Here's how the part is built. I have some questions about the finished solid (model axes, mm). Face numbers are marked on the shaded views. A direction names the side the tool comes from. Round coordinates to 2 decimals unless told otherwise and drop trailing zeros. Write each loop counter-clockwise with the first axis right and the second up, starting at its lowest first coordinate (ties: lowest second). Pieces come first, ordered by that corner, then holes. Notation, with made-up numbers: (69.25, 51) - (78.25, 51) arc R17 ccw to (78.25, 76) - close; hole circle Ø4 at (-39, 19.5). An arc over 180 degrees is marked (long way). Return JSON: item names as keys, results as strings. Group by question number.
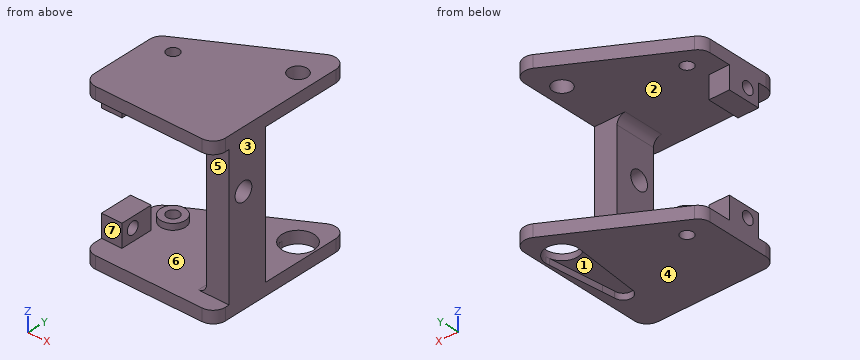
```python
from build123d import *

# Parameters (mm, degrees)
SKETCH1_R           = 1.5
BOSS_EXTRUDE1_DEPTH = 3
SKETCH2_W           = 5
SKETCH2_H           = 8
BOSS_EXTRUDE2_DEPTH = 34
LPATTERN1_COUNT     = 2
LPATTERN1_PITCH     = 37
SKETCH3_W           = 5.5
SKETCH3_H           = 10
BOSS_EXTRUDE4_DEPTH = 34
SKETCH5_W           = 23
SKETCH5_H           = 8
CUT_EXTRUDE1_DEPTH  = 10
CUT_EXTRUDE11_START = -3.7
SKETCH9_R           = 1.5
CUT_EXTRUDE11_DEPTH = 2.2
SKETCH11_R          = 3
SKETCH11_R_2        = 1.5
BOSS_EXTRUDE5_DEPTH = 1.5
SKETCH12_R          = 1.5
CUT_EXTRUDE13_DEPTH = 62.719864532
SKETCH14_R          = 3.9
CUT_EXTRUDE15_DEPTH = 10
SKETCH15_R          = 2.3
CUT_EXTRUDE16_DEPTH = 65.065136212
SKETCH16_R          = 2.25
CUT_EXTRUDE17_DEPTH = 65.065136212
FILLET1_R           = 2


with BuildPart() as part:
    # Sketch1 → Boss-Extrude1 (new body)
    with BuildSketch(Plane.XY):
        with BuildLine():
            Line((-4.5, -2.598076211), (-30.5, -17.60918321))
            ThreePointArc((-30.5, -17.60918321), (-31.598076211, -18.707259422), (-32, -20.207259422))
            Line((-32, -20.207259422), (-32, -35.475208614))
            ThreePointArc((-32, -35.475208614), (-31.121320344, -37.596528958), (-29, -38.475208614))
            Line((-29, -38.475208614), (-3, -38.475208614))
            ThreePointArc((-3, -38.475208614), (-0.878679656, -37.596528958), (0, -35.475208614))
            Line((0, -35.475208614), (0, -5.196152423))
            ThreePointArc((0, -5.196152423), (-1.5, -2.598076211), (-4.5, -2.598076211))
        make_face()
        with Locations((-26, -20.60918321)):
            Circle(SKETCH1_R, mode=Mode.SUBTRACT)
        with Locations((-4.41, -10.598076211)):
            Circle(SKETCH1_R, mode=Mode.SUBTRACT)
    boss_extrude1 = extrude(amount=BOSS_EXTRUDE1_DEPTH)

    # Sketch2 → Boss-Extrude2 (add)
    with BuildSketch(Plane.XY.offset(3)):
        with Locations((-29.5, -29.475208614)):
            Rectangle(SKETCH2_W, SKETCH2_H)
    extrude(amount=BOSS_EXTRUDE2_DEPTH)

    # LPattern1: Boss-Extrude1 ×2
    with Locations(*[(0, 0, i * LPATTERN1_PITCH) for i in range(1, LPATTERN1_COUNT)]):
        add(boss_extrude1)

    # Sketch3 → Boss-Extrude4 (add)
    with BuildSketch(Plane.XY.offset(3)):
        with Locations((-2.75, -29.475208614)):
            Rectangle(SKETCH3_W, SKETCH3_H)
    extrude(amount=BOSS_EXTRUDE4_DEPTH)

    # Sketch5 → Cut-Extrude1 (cut)
    with BuildSketch(Plane.ZY.offset(32)):
        with Locations((20, -29.475208614)):
            Rectangle(SKETCH5_W, SKETCH5_H)
    extrude(amount=-CUT_EXTRUDE1_DEPTH, mode=Mode.SUBTRACT)

    # Sketch9 → Cut-Extrude11 (cut)
    # profile 1 of 2: a face of its own
    with BuildSketch(Plane.XY.offset(3).offset(CUT_EXTRUDE11_START)):
        with BuildLine():
            Line((-8.22147541, -11.42430572), (-6.51, -27.398076211))
            ThreePointArc((-6.51, -27.398076211), (-6.240163927, -28.427882018), (-5.5, -29.193041392))
            Line((-5.5, -29.193041392), (-5.5, -24.475208614))
            Line((-5.5, -24.475208614), (-1.996835615, -24.475208614))
            Line((-1.996835615, -24.475208614), (-0.59852459, -11.42430572))
            Line((-0.59852459, -11.42430572), (-0.51, -10.598076211))
            ThreePointArc((-0.51, -10.598076211), (-4.41, -6.698076211), (-8.31, -10.598076211))
            Line((-8.31, -10.598076211), (-8.22147541, -11.42430572))
        make_face()
        with Locations((-4.41, -10.598076211)):
            Circle(SKETCH9_R, mode=Mode.SUBTRACT)
    # profile 2 of 2: a face of its own
    with BuildSketch(Plane.XY.offset(3).offset(CUT_EXTRUDE11_START)):
        with BuildLine():
            Line((-5.5, -24.475208614), (-5.5, -29.193041392))
            ThreePointArc((-5.5, -29.193041392), (-3.380194193, -29.228240138), (-2.31, -27.398076211))
            Line((-2.31, -27.398076211), (-1.996835615, -24.475208614))
            Line((-1.996835615, -24.475208614), (-5.5, -24.475208614))
        make_face()
    extrude(amount=CUT_EXTRUDE11_DEPTH, mode=Mode.SUBTRACT)

    # Sketch11 → Boss-Extrude5 (add)
    with BuildSketch(Plane.XY.offset(3)):
        with Locations((-26, -20.60918321)):
            Circle(SKETCH11_R)
        with Locations((-26, -20.60918321)):
            Circle(SKETCH11_R_2, mode=Mode.SUBTRACT)
    extrude(amount=BOSS_EXTRUDE5_DEPTH)

    # Sketch12 → Cut-Extrude13 (cut, through all)
    with BuildSketch(Plane(origin=(-27, 0, 0), x_dir=(0, 0, -1), z_dir=(1, 0, 0))):
        with Locations((-34.4, -30.525208614)):
            Circle(SKETCH12_R)
        with Locations((-6, -30.525208614)):
            Circle(SKETCH12_R)
    extrude(amount=-CUT_EXTRUDE13_DEPTH, mode=Mode.SUBTRACT)

    # Sketch14 → Cut-Extrude15 (cut)
    with BuildSketch(Plane(origin=(0, 0, 1.5), x_dir=(-1, 0, 0), z_dir=(0, 0, -1))):
        with Locations(Location((4.41, -10.598076211, 0), (0, 0, 180))):
            Circle(SKETCH14_R)
    extrude(amount=-CUT_EXTRUDE15_DEPTH, mode=Mode.SUBTRACT)

    # Sketch15 → Cut-Extrude16 (cut, through all)
    with BuildSketch(Plane(origin=(0, 0, 0), x_dir=(0, 0, -1), z_dir=(1, 0, 0))):
        with Locations(Location((-25.85, -30.525208614, 0), (0, 0, 90))):
            Circle(SKETCH15_R)
    extrude(amount=-CUT_EXTRUDE16_DEPTH, mode=Mode.SUBTRACT)

    # Sketch16 → Cut-Extrude17 (cut, through all)
    with BuildSketch(Plane.XY.offset(40)):
        with Locations((-4.41, -10.598076211)):
            Circle(SKETCH16_R)
    extrude(amount=-CUT_EXTRUDE17_DEPTH, mode=Mode.SUBTRACT)

    # Fillet1
    fillet1_edges = [part.edges().sort_by_distance(p)[0] for p in [
        (-5.5, -29.475208614, 3),
        (-5.5, -29.475208614, 37),
    ]]
    fillet(fillet1_edges, radius=FILLET1_R)


solid = part.part
```
1) Imagine slicing it at D-D (z = 12). Please give me the cut outline in (x, y).
2) For the marked faces 5, 6 and 7, which set-ups out of +Z, -Z, +X, -X, +Y, -Y let a thin tool reach every point of the face, with its end or its side?
3) If we mould it in two halves opening along X, with no side actions, what happens to the marked faces 1, 2, 3 and 4? For each: released by +X, released by -X, zero draft, split by the parting line, or undercut.
4) I need wall thicknesses on line 1 along Z through (x, y) = (-23.5, -28.5); line 2 along X through (y, z) = (-32, 13); line 3 along X through (y, z) = (-27, 4). Which ranges of each line are inside material? Lowest first, please.
5) Imagine slicing it at C-C (y = -4). Please give me the cut outline in (x, z).
6) Imagine slicing it at B-B (z = 25.85). Please give me the cut outline in (x, y).
7) Imagine slicing it at A-A (z = 34.4). Please give me the cut outline in (x, y).
8) Will these pins go through, and if not, where does the flat tip stop? pin 1 Ø4 at (x, z) = (-3, 17) entering from -Y; pin 2 Ø1.5 at (x, z) = (-28.5, 35.5) entering from +Y; pin 3 Ø1.5 at (y, z) = (-21.5, 5) entering from -X; pin 4 Ø8 at (x, y) = (-15, -6) entering from +Z.
Results found:
{
 "1": {"outline": "(-5.5, -34.48) - (0, -34.48) - (0, -24.48) - (-5.5, -24.48) - close"},
 "2": {"face 5": "+X, -X, -Y", "face 6": "none", "face 7": "-X, -Y"},
 "3": {"face 1": "undercut", "face 2": "undercut", "face 3": "released by +X", "face 4": "zero draft"},
 "4": {"line 1": "z = 0 to 3, 37 to 40", "line 2": "x = -5.5 to 0", "line 3": "x = -32 to -27, -5.77 to 0"},
 "5": {"outline": "(-6.93, 0) - (-0.25, 0) - (-0.25, 3) - (-6.93, 3) - close; (-6.93, 37) - (-0.25, 37) - (-0.25, 40) - (-6.93, 40) - close"},
 "6": {"outline": "(-5.5, -34.48) - (0, -34.48) - (0, -32.83) - (-5.5, -32.83) - close; (-5.5, -28.23) - (0, -28.23) - (0, -24.48) - (-5.5, -24.48) - close"},
 "7": {"outline": "(-32, -33.48) - (-27, -33.48) - (-27, -32.03) - (-32, -32.03) - close; (-32, -29.03) - (-27, -29.03) - (-27, -25.48) - (-32, -25.48) - close; (-5.5, -34.48) - (0, -34.48) - (0, -24.48) - (-5.5, -24.48) - close"},
 "8": {"pin 1": "stops at y = -34.48", "pin 2": "stops at y = -25.48", "pin 3": "stops at x = -28.98", "pin 4": "stops at z = 40"}
}
